```python
from build123d import *

# Parameters (mm, degrees)
SKETCH1_W           = 42
SKETCH1_H           = 90
BOSS_EXTRUDE1_DEPTH = 22
FILLET1_R           = 1
SKETCH2_W           = 38
SKETCH2_H           = 68
CUT_EXTRUDE1_DEPTH  = 20
SKETCH3_W           = 1
SKETCH3_H           = 68
BOSS_EXTRUDE2_DEPTH = 20
SKETCH4_W           = 42
SKETCH4_H           = 88
CUT_EXTRUDE2_DEPTH  = 6.7
CUT_EXTRUDE3_REACH  = 97
SKETCH5_R           = 1.5
SKETCH6_W           = 7
SKETCH6_H           = 5
CUT_EXTRUDE4_DEPTH  = 3
SKETCH7_R           = 2
CUT_EXTRUDE5_DEPTH  = 55.313902456


with BuildPart() as part:
    # Sketch1 → Boss-Extrude1 (new body)
    with BuildSketch(Plane(origin=(0, 0, 0), x_dir=(1, 0, 0), z_dir=(0, 1, 0))):
        Rectangle(SKETCH1_W, SKETCH1_H)
    extrude(amount=BOSS_EXTRUDE1_DEPTH)

    # Fillet1
    fillet1_edges = [part.edges().sort_by_distance(p)[0] for p in [
        (-21, 22, 0),
        (21, 22, 0),
        (-21, 0, 0),
        (21, 0, 0),
    ]]
    fillet(fillet1_edges, radius=FILLET1_R)

    # Sketch2 → Cut-Extrude1 (cut)
    with BuildSketch(Plane(origin=(0, 22, 0), x_dir=(1, 0, 0), z_dir=(0, 1, 0))):
        with Locations((0, -5.7)):
            Rectangle(SKETCH2_W, SKETCH2_H)
    extrude(amount=-CUT_EXTRUDE1_DEPTH, mode=Mode.SUBTRACT)

    # Sketch3 → Boss-Extrude2 (add)
    with BuildSketch(Plane(origin=(0, 2, 0), x_dir=(1, 0, 0), z_dir=(0, 1, 0))):
        with Locations((0, -5.7)):
            Rectangle(SKETCH3_W, SKETCH3_H)
    extrude(amount=BOSS_EXTRUDE2_DEPTH)

    # Sketch4 → Cut-Extrude2 (cut)
    with BuildSketch(Plane(origin=(0, 22, 0), x_dir=(1, 0, 0), z_dir=(0, 1, 0))):
        with Locations((0, 1)):
            Rectangle(SKETCH4_W, SKETCH4_H)
    extrude(amount=-CUT_EXTRUDE2_DEPTH, mode=Mode.SUBTRACT)

    # Sketch5 → Cut-Extrude3 (cut, up to next)
    with BuildSketch(Plane(origin=(0, 0, -45), x_dir=(-1, 0, 0), z_dir=(0, 0, -1)), mode=Mode.PRIVATE) as cut_extrude3_sk1:
        with Locations((-13.5, 3.5)):
            Circle(SKETCH5_R)
    cut_extrude3_tool1 = extrude(cut_extrude3_sk1.sketch, amount=-CUT_EXTRUDE3_REACH, mode=Mode.PRIVATE) & part.part
    add(cut_extrude3_tool1.solids().sort_by_distance((13.5, 3.5, -45))[0], mode=Mode.SUBTRACT)

    # Sketch6 → Cut-Extrude4 (cut)
    with BuildSketch(Plane(origin=(0, 0, -45), x_dir=(-1, 0, 0), z_dir=(0, 0, -1))):
        with Locations((8.5, 12.8)):
            Rectangle(SKETCH6_W, SKETCH6_H)
    extrude(amount=-CUT_EXTRUDE4_DEPTH, mode=Mode.SUBTRACT)

    # Sketch7 → Cut-Extrude5 (cut, through all)
    with BuildSketch(Plane.XZ):
        with Locations(Location((14, -15, 0), (0, 0, 270))):
            Circle(SKETCH7_R)
        with Locations(Location((14, 25, 0), (0, 0, 270))):
            Circle(SKETCH7_R)
        with Locations(Location((-14, 25, 0), (0, 0, 270))):
            Circle(SKETCH7_R)
        with Locations(Location((-14, -15, 0), (0, 0, 270))):
            Circle(SKETCH7_R)
    extrude(amount=-CUT_EXTRUDE5_DEPTH, mode=Mode.SUBTRACT)


solid = part.part
```
Work out the finished part from the listing and answer in its coordinate system (mm). A direction names the side the tool comes from. Coordinates: 2 decimals unless noted, no trailing zeros. Write each loop counter-clockwise with the first axis right and the second up, starting at its lowest first coordinate (ties: lowest second). Pieces come first, ordered by that corner, then holes.
Q1. A cutting plane is placed at C-C, the plane z = -36. Give the vertices of the cut face in (x, y).
Q2. A cutting plane is placed at A-A, the plane z = -15. Give the vertices of the cut face in (x, y).
Q3. Find the intervals of material crossed by line 1 (X direction, y = 10.25, z = -24); line 2 (X direction, y = 0.8, z = 25); line 3 (Z direction, x = -14.5, y = 8.25), in increasing order.
Q4. Which of the six approach directions +Z, -Z, +X, -X, +Y, -Y give full straight-line access (tool end or side, diameter ignored) to faces 1 (the face through (-8, 13, -42)), 2 (the face through (0, 15.3, -18)), 3 (the face through (-19, 9, 6)), 4 (the face through (15, 3.57, -36.77))?
Q5. Determine the mould class of faces 5 (the face through (15.352, 0.986, 26.474)), 6 (the face through (-8, 10.3, -44)), 7 (the face through (21, 6, 1)), 8 (the face through (0, 19, 43)) for opening direction X: released by +X, released by -X, zero draft, split by the parting line, or undercut.
Q6. A cutting plane is placed at D-D, the plane x = -1.5. Give the vertices of the cut face in (y, z).
Q7. A cutting plane is placed at B-B, the plane y = 6. Give the vertices of the cut face in (x, z), then the cut area to 3 significant figures.
Q8. Each of these flat-tipped pins is pushed along its axis until it touches: pin 1 Ø2.5 at (x, y) = (13.5, 3.5) entering from -Z; pin 2 Ø5.5 at (x, y) = (2.5, 19.5) entering from -Z; pin 3 Ø12.5 at (x, z) = (-8.5, -6) entering from +Y; pin 4 Ø2.5 at (x, z) = (14, 25) entering from -Y. Where does it stop, or does it pass through?
Findings below:
1. outline: (-21, 1) arc R1 ccw to (-20, 0) - (20, 0) arc R1 ccw to (21, 1) - (21, 15.3) - (-21, 15.3) - close; hole circle Ø3 at (13.5, 3.5)
2. outline: (-21, 1) arc R1 ccw to (-20, 0) - (-16, 0) - (-16, 2) - (-19, 2) - (-19, 15.3) - (-21, 15.3) - close; (-12, 0) - (12, 0) - (12, 2) - (0.5, 2) - (0.5, 15.3) - (-0.5, 15.3) - (-0.5, 2) - (-12, 2) - close; (16, 0) - (20, 0) arc R1 ccw to (21, 1) - (21, 15.3) - (19, 15.3) - (19, 2) - (16, 2) - close
3. line 1: x = -21 to -19, -0.5 to 0.5, 19 to 21
3. line 2: x = -20.98 to -16, -12 to 12, 16 to 20.98
3. line 3: z = -45 to -28.3, 39.7 to 45
4. face 1: -Z, +Y
4. face 2: -Z, +X, -X, +Y
4. face 3: +Y
4. face 4: -Z
5. face 5: undercut
5. face 6: undercut
5. face 7: released by +X
5. face 8: zero draft
6. outline: (0, -45) - (15.3, -45) - (15.3, -28.3) - (2, -28.3) - (2, 39.7) - (15.3, 39.7) - (15.3, 43) - (22, 43) - (22, 45) - (0, 45) - close
7. outline: (-21, -45) - (21, -45) - (21, 45) - (-21, 45) - close; hole (-19, -28.3) - (-0.5, -28.3) - (-0.5, 39.7) - (-19, 39.7) - close; hole (0.5, -28.3) - (19, -28.3) - (19, 39.7) - (0.5, 39.7) - close
7. area: 1,260 mm2
8. pin 1: stops at z = 39.7
8. pin 2: stops at z = 43
8. pin 3: stops at y = 2
8. pin 4: passes through
